Geometry: final body of the model. Coordinates: model frame, mm. Give positions to 0.01 mm unless a question says otherwise; leave off trailing zeros. Write each loop counter-clockwise with the first axis right and the second up, starting at its lowest first coordinate (ties: lowest second). Pieces come first, ordered by that corner, then holes.
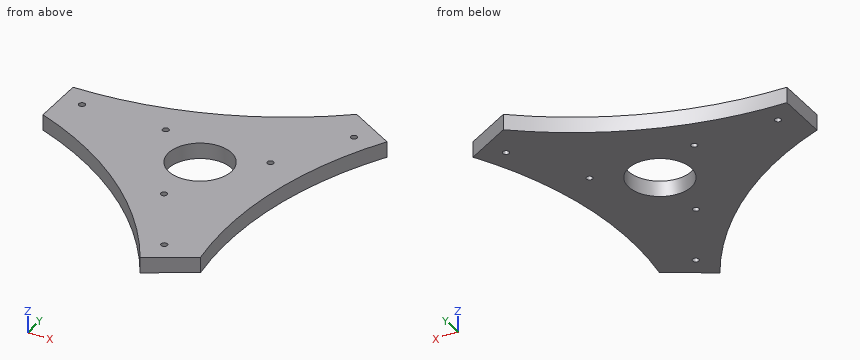
```python
from build123d import *

# Parameters (mm, degrees)
PAD_DEPTH             = 15
SKETCH001_R           = 3
POCKET_DEPTH          = 798.1381594859
POLARPATTERN_COUNT    = 3
POCKET001_DEPTH       = 798.1381594859
POLARPATTERN001_COUNT = 3
SKETCH003_R           = 30
POCKET002_DEPTH       = 15.001


with BuildPart() as part:
    # Sketch → Pad (new body)
    with BuildSketch(Plane.XY):
        Polygon((-150, 0), (-150, 50), (75, 129.9038105677), (118.3012701892, 104.9038105677), (75, -129.9038105677), (31.6987298108, -154.9038105677), align=None)
    extrude(amount=PAD_DEPTH)

    # Sketch001 (on Face8 of Pad) → Pocket (cut, through all)
    with BuildSketch(Plane.XY.offset(15)):
        with Locations((-130, 30)):
            Circle(SKETCH001_R)
        with Locations((-50, 30)):
            Circle(SKETCH001_R)
    pocket = extrude(amount=-POCKET_DEPTH, mode=Mode.SUBTRACT)

    # PolarPattern: Pocket ×3 about axis
    polarpattern_axis = Axis((0, 0, 0), (0, 0, 1))
    for i in range(1, POLARPATTERN_COUNT):
        add(pocket.rotate(polarpattern_axis, i * 360 / POLARPATTERN_COUNT), mode=Mode.SUBTRACT)

    # Sketch002 (on Face5 of PolarPattern) → Pocket001 (cut, through all)
    with BuildSketch(Plane.XY.offset(15)):
        with BuildLine():
            ThreePointArc((-150, 50), (-30.6165642318, 70.5689367266), (75, 129.9038105677))
            Line((-150, 50), (75, 129.9038105677))
        make_face()
    pocket001 = extrude(amount=-POCKET001_DEPTH, mode=Mode.SUBTRACT)

    # PolarPattern001: Pocket001 ×3 about axis
    polarpattern001_axis = Axis((0, 0, 0), (0, 0, 1))
    for i in range(1, POLARPATTERN001_COUNT):
        add(pocket001.rotate(polarpattern001_axis, i * 360 / POLARPATTERN001_COUNT), mode=Mode.SUBTRACT)

    # Sketch003 (on Face5 of PolarPattern001) → Pocket002 (cut, through all)
    with BuildSketch(Plane.XY.offset(15)):
        Circle(SKETCH003_R)
    extrude(amount=-POCKET002_DEPTH, mode=Mode.SUBTRACT)


solid = part.part
```
Item 1: Line query: L1, parallel to Y at x = -132.5, z = 13.75; L2, parallel to X at y = -15, z = 12; L3, parallel to Y at x = 0.5, z = 14.25. Output: solid intervals per line, ascending.
Found:
L1: y = -7.22 to 28.34, 31.66 to 50.43
L2: x = -116.11 to -25.98, 25.98 to 75.33
L3: y = -109.4 to -60.91, -55.69 to -30, 30 to 83.3
Item 2: Section B-B, the plane x = -83.5. Return the cut outline in (y, z), plus the area to 3 significant figures.
Found:
outline: (-33.73, 0) - (56.25, 0) - (56.25, 15) - (-33.73, 15) - close
area: 1,350 mm2
Item 3: Section A-A, the plane z = 10. Return the cut outline in (x, y).
Found:
outline: (-150, 0) arc R356.74 cw to (31.7, -154.9) - (75, -129.9) arc R356.74 cw to (118.3, 104.9) - (75, 129.9) arc R356.74 cw to (-150, 50) - close; hole circle Ø6 at (-130, 30); hole circle Ø6 at (-50, 30); hole circle Ø60 at (0, 0); hole circle Ø6 at (-0.98, -58.3); hole circle Ø6 at (39.02, -127.58); hole circle Ø6 at (50.98, 28.3); hole circle Ø6 at (90.98, 97.58)
Item 4: Pin query (flat end, axial travel): pin 1 Ø4 at (x, z) = (-36, 1.5) entering from +Y; pin 2 Ø4 at (x, z) = (-1.5, 7.5) entering from -Y; pin 3 Ø5 at (y, z) = (40, 1.5) entering from +X. Return the tip coordinate at first contact, or that it passes through.
Found:
pin 1: stops at y = 69.39
pin 2: stops at y = -109.4
pin 3: stops at x = 89.88
Item 5: Section C-C, the plane y = 39.5. Return the cut outline in (x, z).
Found:
outline: (-150, 0) - (88.87, 0) - (88.87, 15) - (-150, 15) - close
